The model under review builds one solid part; all positions refer to its coordinate system, in mm. Face numbers are marked on the shaded views. A direction names the side the tool comes from. Coordinates: 2 decimals unless noted, no trailing zeros. Order: outer loops, then holes, each group sorted by start corner. A loop starts at its lowest first (then second) coordinate and runs counter-clockwise, first axis right, second up. Notation, with made-up numbers: (23.25, 47.5) -> (52.25, 47.5) arc R16 cw to (52.25, 75.5) -> close; hole circle Ø8 at (30, -32.5). An arc over 180 degrees is marked (long way). Put each result on its own line as item: value.
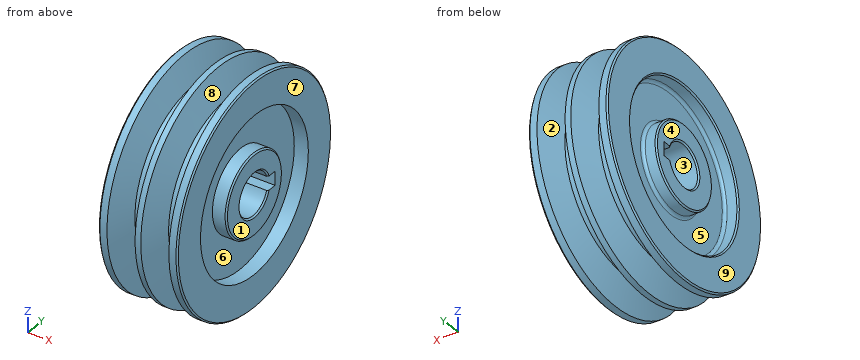
from build123d import *

# Parameters (mm, degrees)
CHAMFER1_SIZE      = 0.5
CHAMFER2_SIZE      = 0.5
FILLET2_R          = 1
CUT_EXTRUDE1_DEPTH = 64.118935352


with BuildPart() as part:
    # Sketch1 → Revolve1 (revolve)
    with BuildSketch(Plane(origin=(0, 0, 0), x_dir=(1, 0, 0), z_dir=(0, 1, 0))):
        Polygon((-14, 40), (-14, 28), (-9, 28), (-9, 14.5), (-14, 14.5), (-14, 7.5), (14, 7.5), (14, 14.5), (9, 14.5), (9, 28), (14, 28), (14, 40), (11, 40), (7.942693185, 30), (4.057306815, 30), (1, 40), (-1, 40), (-4.057306815, 30), (-7.942693185, 30), (-11, 40), align=None)
    revolve(axis=Axis((0, 0, 0), (-1, 0, 0)))

    # Chamfer1
    chamfer1_edges = [part.edges().sort_by_distance(p)[0] for p in [
        (14, 0, 7.5),
        (14, 0, 14.5),
        (14, 0, 40),
    ]]
    chamfer(chamfer1_edges, length=CHAMFER1_SIZE)

    # Chamfer2
    chamfer2_edges = [part.edges().sort_by_distance(p)[0] for p in [
        (-14, 0, 40),
        (-14, 0, 28),
        (-14, 0, 14.5),
        (-14, 0, 7.5),
    ]]
    chamfer(chamfer2_edges, length=CHAMFER2_SIZE)

    # Fillet2
    fillet2_edges = [part.edges().sort_by_distance(p)[0] for p in [
        (-9, 0, 28),
        (-9, 0, 14.5),
    ]]
    fillet(fillet2_edges, radius=FILLET2_R)

    # Sketch2 → Cut-Extrude1 (cut, through all)
    with BuildSketch(Plane(origin=(14, 0, 0), x_dir=(0, 0, -1), z_dir=(1, 0, 0))):
        Polygon((-2.5, 7.5), (-2.5, 5.832980878), (2.5, 5.832980878), (2.5, 7.5), (2.5, 10.7), (-2.5, 10.7), align=None)
    extrude(amount=-CUT_EXTRUDE1_DEPTH, mode=Mode.SUBTRACT)


solid = part.part
Item 1: For pin 1 Ø1.5 at (x, z) = (0, 0) entering from -Y; pin 2 Ø3 at (x, z) = (11, -12) entering from +Y; pin 3 Ø13.5 at (y, z) = (0, 0) entering from +X; pin 4 Ø1.5 at (x, z) = (-1, -6) entering from +Y, all flat-tipped, find the tip position at first contact; note any pin that passes through.
Answers below:
pin 1: y = -40
pin 2: y = 38.6
pin 3: through
pin 4: y = 39.65
Item 2: Consider section C-C on x = 2.5. Write out the cut boundary in (y, z).
Answers below:
outline: circle Ø70.19 at (0, 0); hole (7.07, -2.5) -> (10.7, -2.5) -> (10.7, 2.5) -> (7.07, 2.5) arc R7.5 ccw (long way) to start
Item 3: Consider section B-B on z = -33.5. Count the separate pieces of the cut face and the enclosed holes in it, and give its area (3 significant figures).
Answers below:
separate pieces: 3
enclosed holes: 0
area: 576 mm^2
Item 4: For the marked faces 5, 6, 7, 8 and 9, list the 3-axis set-ups (+Z, -Z, +X, -X, +Y, -Y) from which the entire face can be reached by the end or side of a thin tool; tool diameter is ignored.
Answers below:
face 5: -X
face 6: +X
face 7: +Z, -Z, +X, +Y, -Y
face 8: none
face 9: +Z, -Z, -X, +Y, -Y
Item 5: Consider section A-A on x = 10. Write out the cut boundary in (y, z).
Answers below:
outline: circle Ø73.46 at (0, 0); circle Ø29 at (0, 0); hole circle Ø56 at (0, 0); hole (7.07, -2.5) -> (10.7, -2.5) -> (10.7, 2.5) -> (7.07, 2.5) arc R7.5 ccw (long way) to start
Item 6: For line 1 (Z direction, x = -11.6, y = 0); line 2 (X direction, y = -25, z = -20); line 3 (Y direction, x = -5.5, z = 0), list the stretches that pass through material, from the lowest coordinate up. Write a range as from..to.
Answers below:
line 1: -40..-28, -14.5..-7.5, 7.5..14.5, 28..40
line 2: -14..-8.56, -3.44..3.44, 8.56..14
line 3: -30..-7.5, 10.7..30
Item 7: Mouldability with a two-part tool opening along X and no side actions: class the marked faces 1, 2, 3 and 4 as +X half, -X half, draft (parallel to the pull), parting line (faces both ways), or undercut.
Answers below:
face 1: +X half
face 2: undercut
face 3: draft
face 4: -X half
